The model under review builds one solid part; all positions refer to its coordinate system, in mm. Face numbers are marked on the shaded views. Coordinates: 2 decimals unless noted, no trailing zeros. Write each loop counter-clockwise with the first axis right and the second up, starting at its lowest first coordinate (ties: lowest second). Pieces come first, ordered by that corner, then holes. Notation, with made-up numbers: (-15.5, 72) - (6.5, 72) arc R15 ccw to (6.5, 90) - close; hole circle Ø3 at (87, 31). An arc over 180 degrees is marked (long way). Return JSON: item names as keys, results as strings. Group by question number.
(1) Draft analysis for pull direction Y (two halves, no side actions). For the marked faces 1 and 2, state which applies: released by +Y, released by -Y, zero draft, split by the parting line, or undercut.
(2) We need section D-D on y = 20.5. State the section outline as (x, z) points, then the cut area to 3 significant figures.
(3) We need section A-A on x = 0. State the section outline as (y, z) points.
(4) To check wall thickness, follow L1, parallel to Y at x = -1, z = 90.5; L2, parallel to Z at x = 0, y = 23.5; L3, parallel to X at y = -5, z = 88. State the ranges of each line that lie inside material, in increasing order. Write a range as from..to.
(5) For pin 1 Ø1.9 at (y, z) = (0, 115) entering from +X; pin 2 Ø3 at (x, z) = (16.5, 64.5) entering from -Y; pin 3 Ø10 at (x, z) = (16, 21.5) entering from -Y; pin 4 Ø4 at (x, z) = (0, 115) entering from +Y, all flat-tipped, find the tip position at first contact; note any pin that passes through.
(6) We need section C-C on z = 115. State the section outline as (x, y) points, then the cut area to 3 significant figures.
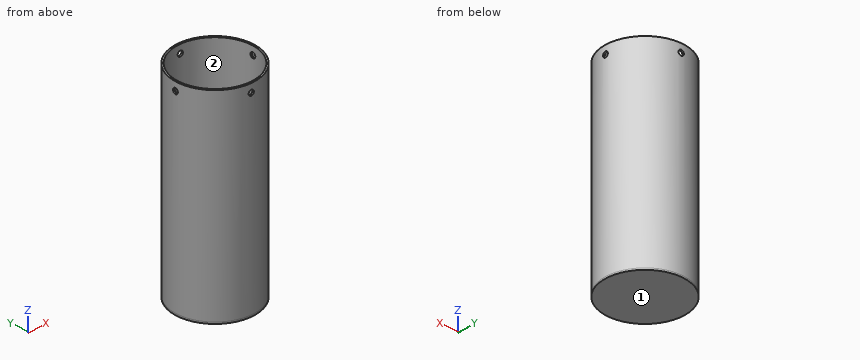
```python
from build123d import *

# Parameters (mm, degrees)
SKETCH1_R               = 24.016
SKETCH1_R_2             = 23
EXTRUDE_THIN1_DEPTH     = 120
BOSS_EXTRUDE1_START     = 1.016
SKETCH2_R               = 24.016
BOSS_EXTRUDE1_DEPTH     = 1.016
CUT_EXTRUDE1_DEPTH      = 125.713818448
CUT_EXTRUDE1_DEPTH_BACK = 125.713818448
SKETCH3_R               = 1.6
CUT_EXTRUDE2_DEPTH      = 125.713818587
CUT_EXTRUDE2_DEPTH_BACK = 125.713818587
SKETCH4_R               = 1.6


with BuildPart() as part:
    # Sketch1 → Extrude-Thin1 (new body)
    with BuildSketch(Plane.XY):
        Circle(SKETCH1_R)
        Circle(SKETCH1_R_2, mode=Mode.SUBTRACT)
    extrude(amount=EXTRUDE_THIN1_DEPTH)

    # Sketch2 → Boss-Extrude1 (add)
    with BuildSketch(Plane(origin=(0, 0, 0), x_dir=(-1, 0, 0), z_dir=(0, 0, -1)).offset(BOSS_EXTRUDE1_START)):
        Circle(SKETCH2_R)
    extrude(amount=-BOSS_EXTRUDE1_DEPTH)

    # Sketch3 → Cut-Extrude1 (cut, two sides: drawn at the far end of the back side and taken through both)
    with BuildSketch(Plane(origin=(0, 0, 0), x_dir=(1, 0, 0), z_dir=(0, 1, 0)).offset(-CUT_EXTRUDE1_DEPTH_BACK)):
        with Locations(Location((0, -115, 0), (0, 0, 270))):
            Circle(SKETCH3_R)
    extrude(amount=CUT_EXTRUDE1_DEPTH + CUT_EXTRUDE1_DEPTH_BACK, mode=Mode.SUBTRACT)

    # Sketch4 → Cut-Extrude2 (cut, two sides: drawn at the far end of the back side and taken through both)
    with BuildSketch(Plane(origin=(0, 0, 0), x_dir=(0, 0, -1), z_dir=(1, 0, 0)).offset(-CUT_EXTRUDE2_DEPTH_BACK)):
        with Locations((-115, 0)):
            Circle(SKETCH4_R)
    extrude(amount=CUT_EXTRUDE2_DEPTH + CUT_EXTRUDE2_DEPTH_BACK, mode=Mode.SUBTRACT)


solid = part.part
```
Ans:
{
 "1": {"face 1": "zero draft", "face 2": "undercut"},
 "2": {"outline": "(-12.51, -1.02) - (12.51, -1.02) - (12.51, 120) - (10.43, 120) - (10.43, 0) - (-10.43, 0) - (-10.43, 120) - (-12.51, 120) - close", "area": "525 mm²"},
 "3": {"outline": "(-24.02, -1.02) - (24.02, -1.02) - (24.02, 113.4) - (23, 113.4) - (23, 0) - (-23, 0) - (-23, 113.4) - (-24.02, 113.4) - close; (-24.02, 116.6) - (-23, 116.6) - (-23, 120) - (-24.02, 120) - close; (23, 116.6) - (24.02, 116.6) - (24.02, 120) - (23, 120) - close"},
 "4": {"L1": "-24..-22.98, 22.98..24", "L2": "-1.02..113.4, 116.6..120", "L3": "-23.49..-22.45, 22.45..23.49"},
 "5": {"pin 1": "through", "pin 2": "y = -18.76", "pin 3": "y = -21.35", "pin 4": "y = 24.02"},
 "6": {"outline": "(-23.96, -1.6) arc R24.02 ccw to (-1.6, -23.96) - (-1.6, -22.94) arc R23 cw to (-22.94, -1.6) - close; (-23.96, 1.6) - (-22.94, 1.6) arc R23 cw to (-1.6, 22.94) - (-1.6, 23.96) arc R24.02 ccw to start; (1.6, -23.96) arc R24.02 ccw to (23.96, -1.6) - (22.94, -1.6) arc R23 cw to (1.6, -22.94) - close; (1.6, 22.94) arc R23 cw to (22.94, 1.6) - (23.96, 1.6) arc R24.02 ccw to (1.6, 23.96) - close", "area": "137 mm²"}
}
